Here's how the part is built. I have some questions about the finished solid (model axes, mm). Face numbers are marked on the shaded views. Give positions to 0.01 mm unless a question says otherwise; leave off trailing zeros. Loops run counter-clockwise (first coordinate to the right, second up) from the corner with the lowest first, then second, coordinate; pieces in that order, holes last. Notation, with made-up numbers: (11, -29) - (62, -29) arc R12 ccw to (62, -9) - close; hole circle Ø1 at (78.5, 87.25). An arc over 180 degrees is marked (long way). Use one line per item in the form item = value.
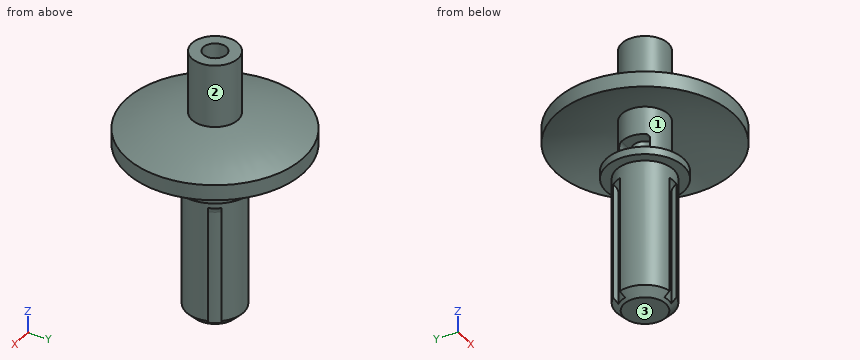
from build123d import *

# Parameters (mm, degrees)
F0_R        = 3.7
F1_DEPTH    = 17.5
F3_DEPTH    = 16
F4_T2_ANGLE = 116.4603484981
F4_T4_ANGLE = 116.4603484981
F4_T6_ANGLE = 116.4603484981
F5_T2_ANGLE = 176.2935685117
F5_T4_ANGLE = 176.2935685117
F5_T6_ANGLE = 58.1290115734
F5_T8_ANGLE = 118.1404591149
F6_R        = 5
F7_DEPTH    = 1
F8_R        = 3
F9_DEPTH    = 16
F14_DEPTH   = 25
F15_R       = 1.5
F16_DEPTH   = 25


# Not quite as in the source:
# - a fillet or chamfer that OpenCascade refuses, or shapes differently, is made with other operations: its cross-section is extruded or revolved along the edge and cut away or added


with BuildPart() as f1:
    # F0 (on Top) → F1 (new body)
    with BuildSketch(Plane.XY):
        Circle(F0_R)
    extrude(amount=-F1_DEPTH)

    # F2 (on face) → F3 (cut)
    with BuildSketch(Plane(origin=(0, 0, -17.5), x_dir=(1, 0, 0), z_dir=(0, 0, -1))):
        with BuildLine():
            ThreePointArc((-2.1852734229, -2.1276936027), (-2.6413774815, -1.525), (-2.9352734229, -0.8286554971))
            Line((-2.9352734229, -0.8286554971), (-3.5127738924, -1.1620755486))
            ThreePointArc((-3.5127738924, -1.1620755486), (-3.204293994, -1.85), (-2.7627738924, -2.4611136543))
            Line((-2.7627738924, -2.4611136543), (-2.1852734229, -2.1276936027))
        make_face()
        with BuildLine():
            Line((-0.75, 3.6231892029), (-0.75, 2.9563490998))
            ThreePointArc((-0.75, 2.9563490998), (0, 3.05), (0.75, 2.9563490998))
            Line((0.75, 2.9563490998), (0.75, 3.6231892029))
            ThreePointArc((0.75, 3.6231892029), (0, 3.7), (-0.75, 3.6231892029))
        make_face()
        with BuildLine():
            Line((2.1852734229, -2.1276936027), (2.7627738924, -2.4611136543))
            ThreePointArc((2.7627738924, -2.4611136543), (3.204293994, -1.85), (3.5127738924, -1.1620755486))
            Line((3.5127738924, -1.1620755486), (2.9352734229, -0.8286554971))
            ThreePointArc((2.9352734229, -0.8286554971), (2.6413774815, -1.525), (2.1852734229, -2.1276936027))
        make_face()
    extrude(amount=-F3_DEPTH, mode=Mode.SUBTRACT)

    # F4: fillet of radius 1 on 3 edges, made by hand

    # F4_s1 → F4_t2 (revolve)
    with BuildSketch(Plane(origin=(0, 0, 0), x_dir=(0, 0, 1), z_dir=(-0.473014829, -0.8810544657, 0))):
        with BuildLine():
            ThreePointArc((-1.5, -3.7), (-1.8666619872, -3.2284161637), (-2.4367496998, -3.05))
            Line((-2.4367496998, -3.05), (-1.5, -3.05))
            Line((-1.5, -3.05), (-1.5, -3.7))
        make_face()
    revolve(axis=Axis((0, 0, -1.5), (0, 0, 1)), revolution_arc=F4_T2_ANGLE)

    # F4_s3 → F4_t4 (revolve)
    with BuildSketch(Plane(origin=(0, 0, 0), x_dir=(0, 0, 1), z_dir=(-0.526508135, 0.8501700911, 0))):
        with BuildLine():
            ThreePointArc((-1.5, -3.7), (-1.8666619872, -3.2284161637), (-2.4367496998, -3.05))
            Line((-2.4367496998, -3.05), (-1.5, -3.05))
            Line((-1.5, -3.05), (-1.5, -3.7))
        make_face()
    revolve(axis=Axis((0, 0, -1.5), (0, 0, 1)), revolution_arc=F4_T4_ANGLE)

    # F4_s5 → F4_t6 (revolve)
    with BuildSketch(Plane(origin=(0, 0, 0), x_dir=(0, 0, 1), z_dir=(0.9995229639, 0.0308843746, 0))):
        with BuildLine():
            ThreePointArc((-1.5, -3.7), (-1.8666619872, -3.2284161637), (-2.4367496998, -3.05))
            Line((-2.4367496998, -3.05), (-1.5, -3.05))
            Line((-1.5, -3.05), (-1.5, -3.7))
        make_face()
    revolve(axis=Axis((0, 0, -1.5), (0, 0, 1)), revolution_arc=F4_T6_ANGLE)

    # F5: chamfer of 1 on 4 edges, made by hand

    # F5_s1 → F5_t2 (revolve, cut)
    with BuildSketch(Plane(origin=(0, 0, 0), x_dir=(0, 0, 1), z_dir=(0.8494028952, 0.5277449399, 0))):
        Polygon((-16.5, -3.7), (-17.5, -2.7), (-17.5, -3.7), align=None)
    revolve(axis=Axis((0, 0, -17.5), (0, 0, 1)), revolution_arc=F5_T2_ANGLE, mode=Mode.SUBTRACT)

    # F5_s3 → F5_t4 (revolve, cut)
    with BuildSketch(Plane(origin=(0, 0, 0), x_dir=(0, 0, 1), z_dir=(0.032339077, -0.9994769553, 0))):
        Polygon((-16.5, -3.7), (-17.5, -2.7), (-17.5, -3.7), align=None)
    revolve(axis=Axis((0, 0, -17.5), (0, 0, 1)), revolution_arc=F5_T4_ANGLE, mode=Mode.SUBTRACT)

    # F5_s5 → F5_t6 (revolve, cut)
    with BuildSketch(Plane.XZ):
        Polygon((3.7, -16.5), (2.7, -17.5), (3.7, -17.5), align=None)
    revolve(axis=Axis((0, 0, -17.5), (0, 0, 1)), revolution_arc=F5_T6_ANGLE, mode=Mode.SUBTRACT)

    # F5_s7 → F5_t8 (revolve, cut)
    with BuildSketch(Plane(origin=(0, 0, 0), x_dir=(0, 0, 1), z_dir=(-0.8817940435, 0.471634673, 0))):
        Polygon((-16.5, -3.7), (-17.5, -2.7), (-17.5, -3.7), align=None)
    revolve(axis=Axis((0, 0, -17.5), (0, 0, 1)), revolution_arc=F5_T8_ANGLE, mode=Mode.SUBTRACT)

    # F6 (on face) → F7 (join)
    with BuildSketch(Plane.XY):
        Circle(F6_R)
    extrude(amount=F7_DEPTH)

    # F8 (on face) → F9 (join)
    with BuildSketch(Plane.XY.offset(1)):
        Circle(F8_R)
    extrude(amount=F9_DEPTH)

    # F10 (on Right) → F12 (revolve)
    with BuildSketch(Plane.YZ):
        with BuildLine():
            Line((0, 8), (0, 9))
            ThreePointArc((0, 9), (-5.863059775, 8.4214977538), (-11.5, 6.708302005))
            Line((-11.5, 6.708302005), (-11.5, 4.708302005))
            ThreePointArc((-11.5, 4.708302005), (-5.9157247408, 6.9331331941), (0, 8))
        make_face()
    revolve(axis=Axis((0, 0, 8.2032438368), (0, 0, 1)))

    # F13 (on Right) → F14 (cut)
    with BuildSketch(Plane.YZ):
        with BuildLine():
            ThreePointArc((2, 3.5), (1.8535533906, 3.8535533906), (1.5, 4))
            Line((1.5, 4), (-1.5, 4))
            ThreePointArc((-1.5, 4), (-1.8535533906, 3.8535533906), (-2, 3.5))
            Line((-2, 3.5), (-2, 2.5))
            ThreePointArc((-2, 2.5), (-1.8535533906, 2.1464466094), (-1.5, 2))
            Line((-1.5, 2), (1.5, 2))
            ThreePointArc((1.5, 2), (1.8535533906, 2.1464466094), (2, 2.5))
            Line((2, 2.5), (2, 3.5))
        make_face()
    extrude(amount=-F14_DEPTH, mode=Mode.SUBTRACT)

    # F15 (on face) → F16 (cut)
    with BuildSketch(Plane.XY.offset(17)):
        Circle(F15_R)
    extrude(amount=-F16_DEPTH, mode=Mode.SUBTRACT)


solid = f1.part
(1) If we section it at C-C (z = 5.5): Give the number of separate pieces and of enclosed holes in the cut face, plus the area to 3 significant figures.
Geometry says:
separate_pieces = 2
enclosed_holes = 2
area = 131 mm²
(2) If we section it at A-A (z = 15.5): List the corners of the cut face in (x, y) for me, plus the area to 3 significant figures.
Geometry says:
outline = circle Ø6 at (0, 0); hole circle Ø3 at (0, 0)
area = 21.2 mm²
(3) Thinking about a two-plate mould opening in X: for the marked faces 1, 2 and 3, which applies, pulls with the +X half, pulls with the -X half, needs draft (parallel to the pull), parting line crosses it, or undercut?
Geometry says:
face_1 = undercut
face_2 = parting line crosses it
face_3 = needs draft
(4) For P1, Ø12, axis at y = -8.5, z = 1, coming from the +X side; P2, Ø0.7, axis at y = -3.5, z = -9.5, coming from the -X side; P3, Ø10, axis at x = 8.5, y = 7.5, coming from the -Z side; P4, Ø1, axis at x = -5.5, z = -14, coming from the +Y side, each with a flat end and sliding along its axis, tell me the tip position at first contact or that it passes through.
Geometry says:
P1 = 10.86
P2 = -1.94
P3 = 4.71
P4 = through
(5) If I drill on probe 1 along Y at (x, z) = (0, -2.5); probe 2 along X at (y, z) = (0, -0.5); probe 3 along X at (y, z) = (0, 5.5), over which ranges is the centre line in solid material (lowest first)?
Geometry says:
probe_1 = -3.05 to -1.5, 1.5 to 3.7
probe_2 = -3.7 to -1.5, 1.5 to 3.7
probe_3 = -11.5 to -9.86, -3 to -1.5, 1.5 to 3, 9.86 to 11.5
(6) If we section it at B-B (z = -11): List the corners of the cut face in (x, y) for me, plus the area to 3 significant figures.
Geometry says:
outline = (-3.51, 1.16) arc R3.7 ccw to (-0.75, -3.62) - (-0.75, -2.96) arc R3.05 ccw to (0.75, -2.96) - (0.75, -3.62) arc R3.7 ccw to (3.51, 1.16) - (2.94, 0.83) arc R3.05 ccw to (2.19, 2.13) - (2.76, 2.46) arc R3.7 ccw to (-2.76, 2.46) - (-2.19, 2.13) arc R3.05 ccw to (-2.94, 0.83) - close
area = 40.1 mm²
